Source: CAD feature listing. Evaluate the final solid. Frame: model axes, mm. Face numbers are marked on the shaded views. Round coordinates to 2 decimals unless told otherwise and drop trailing zeros. Order: outer loops, then holes, each group sorted by start corner. A loop starts at its lowest first (then second) coordinate and runs counter-clockwise, first axis right, second up. Notation, with made-up numbers: (85.5, 74) -> (107.5, 74) arc R15 cw to (107.5, 80) -> close; hole circle Ø8 at (52, -5.5). An arc over 180 degrees is marked (long way). Answer as CSV lines item,"result". Start each with the question number.
(1) Contact query for a flat-ended pin moving along its axis: P1, Ø2, axis at x = 94, y = 453, coming from the -Z side. Output: stop coordinate, or through.
(2) Line query: line 1 along Y through (x, z) = (292, 16.5); line 2 along X through (y, z) = (-463.5, -2); line 3 along X through (y, z) = (23.5, 66). Output: solid intervals per line, ascending. Write a range as from..to.
(3) Section query B-B (x = -54). Output: boundary loops of the cut face in (y, z).
(4) Section query C-C (y = -467.5). Output: boundary loops of the cut face in (x, z), plus the area to 3 significant figures.
(5) Pull-direction query (X, two-part tool) for the marked faces 1 and 2; classes: +X half, -X half, draft (parallel to the pull), parting line (faces both ways), or undercut.
(6) Section query A-A (z = -2.5). Output: boundary loops of the cut face in (x, y).
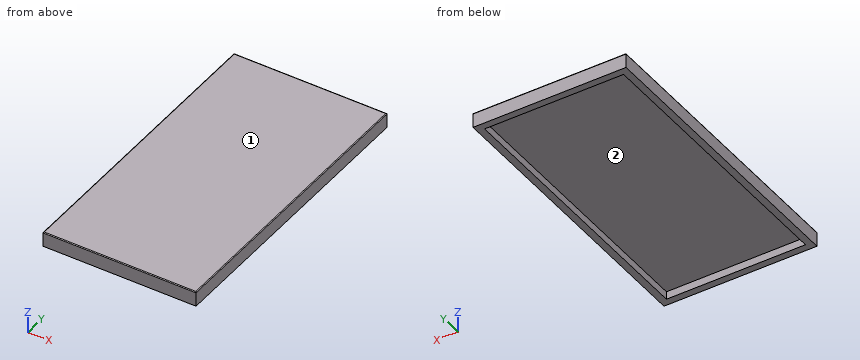
```python
from build123d import *

# Parameters (mm, degrees)
F0_W        = 980
F0_H        = 1890
F1_DEPTH    = 70
F2_R        = 5
F3_W        = 980
F3_H        = 1890
F1_FACE_W   = 980
F1_FACE_H   = 1890
F1_FACE_W_2 = 970
F1_FACE_H_2 = 1880
F4_DEPTH    = 25
F5_W        = 890
F5_H        = 1800
F6_DEPTH    = 50


with BuildPart() as f1:
    # F0 (on Top) → F1 (new body)
    with BuildSketch(Plane.XY):
        Rectangle(F0_W, F0_H)
    extrude(amount=F1_DEPTH)

    # F2
    f2_edges = [f1.edges().sort_by_distance(p)[0] for p in [
        (0, 945, 70),
        (-490, 0, 70),
        (0, -945, 70),
        (490, 0, 70),
    ]]
    fillet(f2_edges, radius=F2_R)

    # F3 (on face) + F1_face (on face) → F4 (join)
    with BuildSketch(Plane(origin=(0, 0, 0), x_dir=(1, 0, 0), z_dir=(0, 0, -1))):
        Rectangle(F3_W, F3_H)
    with BuildSketch(Plane(origin=(0, 0, 0), x_dir=(1, 0, 0), z_dir=(0, 0, -1))):
        Rectangle(F1_FACE_W, F1_FACE_H)
        Rectangle(F1_FACE_W_2, F1_FACE_H_2)
    extrude(amount=F4_DEPTH)

    # F5 (on face) → F6 (cut)
    with BuildSketch(Plane(origin=(0, 0, -25), x_dir=(1, 0, 0), z_dir=(0, 0, -1))):
        Rectangle(F5_W, F5_H)
    extrude(amount=-F6_DEPTH, mode=Mode.SUBTRACT)


solid = f1.part
```
Answer block:
1,P1,"z = 25"
2,line 1,"-945..-900, 900..945"
2,line 2,"-490..-445, 445..490"
2,line 3,"-489.9..489.9"
3,outline,"(-945, -25) -> (-900, -25) -> (-900, 25) -> (900, 25) -> (900, -25) -> (945, -25) -> (945, 65) arc R5 ccw to (940, 70) -> (-940, 70) arc R5 ccw to (-945, 65) -> close"
4,outline,"(-490, -25) -> (-445, -25) -> (-445, 25) -> (445, 25) -> (445, -25) -> (490, -25) -> (490, 65) arc R5 ccw to (485, 70) -> (-485, 70) arc R5 ccw to (-490, 65) -> close"
4,area,"48,600 mm2"
5,face 1,"draft"
5,face 2,"undercut"
6,outline,"(-490, -945) -> (490, -945) -> (490, 945) -> (-490, 945) -> close; hole (-445, -900) -> (445, -900) -> (445, 900) -> (-445, 900) -> close"
